The figure shows three views and two pictorial views of one solid part (mm, origin at its lowest corner). Answer the questions. Coordinates: 2 decimals unless noted, no trailing zeros. Loops run counter-clockwise (first coordinate to the right, second up) from the corner with the lowest first, then second, coordinate; pieces in that order, holes last. Notation, with made-up numbers: M 66,72 L 90,72 A19 ccw 90,94 Z; hole C 20,23.5 d10. An arc over 180 degrees is marked long. One line per item, written item: value. Start each with the question number.
1. Consider probe 1 along Z at (x, y) = (22, 7.5). Determine where the line is inside the solid, lowest interval first.
2. Flat-ended cylindrical pins translate along their axes: pin 1 (5 mm diameter, centred on x = 40, z = 42.5, fed in from -Y); pin 2 (3 mm diameter, centred on x = 31, y = 39.5, fed in from -Z). Find the tip coordinate at first contact, or state that the pin passes through.
3. The part is cut by section A-A (x = 21). Write down the section's boundary in (y, z).
4. Determine the mould class of the marked faces 1, 2 and 3 for opening direction X: +X half, -X half, draft (parallel to the pull), parting line (faces both ways), or undercut.
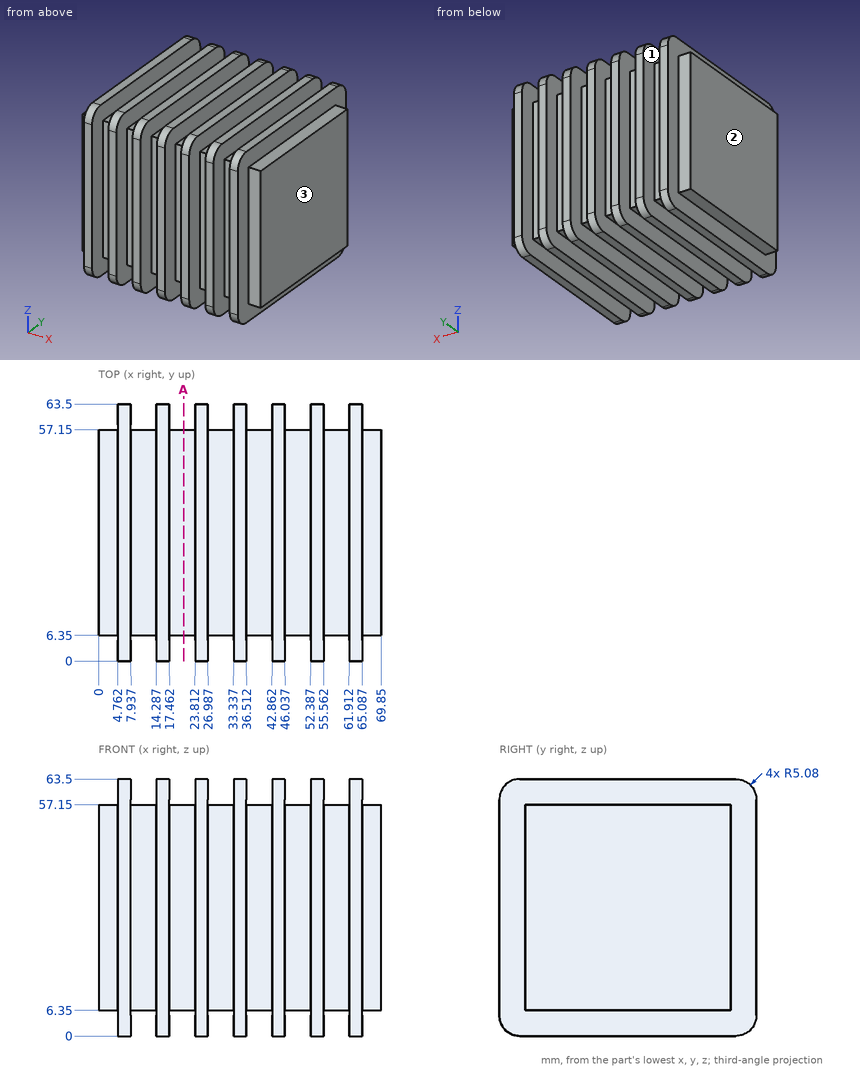
Answer block:
1. probe 1: z = 6.35 to 57.15
2. pin 1: stops at y = 6.35
2. pin 2: stops at z = 6.35
3. outline: M 6.35,6.35 L 57.15,6.35 L 57.15,57.15 L 6.35,57.15 Z
4. face 1: undercut
4. face 2: -X half
4. face 3: +X half
